Geometry check sheet. Reference: the model listing, model coordinates, mm. Face numbers are marked on the shaded views. A direction names the side the tool comes from. Coordinates: 2 decimals unless noted, no trailing zeros. Write each loop counter-clockwise with the first axis right and the second up, starting at its lowest first coordinate (ties: lowest second). Pieces come first, ordered by that corner, then holes. Notation, with made-up numbers: (-28, 45) - (-3, 45) arc R31 cw to (-3, 83) - close; hole circle Ø8 at (35.25, 49.25). An arc over 180 degrees is marked (long way). Answer as a JSON object with one key per item and string values. Group by question number.
from build123d import *

# Parameters (mm, degrees)
SKETCH1_R               = 5
BOSS_EXTRUDE1_DEPTH     = 22
FILLET1_R               = 1
FILLET2_R               = 10
SKETCH3_W               = 18
SKETCH3_H               = 10
CUT_EXTRUDE2_DEPTH      = 45
CUT_EXTRUDE2_DEPTH_BACK = 46


with BuildPart() as part:
    # Sketch1 → Boss-Extrude1 (new body)
    with BuildSketch(Plane(origin=(0, 0, 0), x_dir=(1, 0, 0), z_dir=(0, 1, 0))):
        with BuildLine():
            Line((44, 17), (35, 26))
            Line((35, 26), (25, 26))
            Line((25, 26), (5, 20.641016151))
            Line((5, 20.641016151), (-15, 26))
            Line((-15, 26), (-25, 26))
            Line((-25, 26), (-44.391127187, -9.608765584))
            ThreePointArc((-44.391127187, -9.608765584), (-38.766232585, -7.154608585), (-35, -12))
            ThreePointArc((-35, -12), (-36.464466094, -15.535533906), (-40, -17))
            Line((-40, -17), (-26.36195996, -17))
            Line((-26.36195996, -17), (-13.660254038, 5))
            ThreePointArc((-13.660254038, 5), (-10, 8.660254038), (-5, 10))
            Line((-5, 10), (5, 10))
            ThreePointArc((5, 10), (10, 8.660254038), (13.660254038, 5))
            Line((13.660254038, 5), (25.784609691, -16))
            Line((25.784609691, -16), (44, -16))
            Line((44, -16), (44, -4))
            Line((44, -4), (39.5, 0.5))
            Line((39.5, 0.5), (44, 5))
            Line((44, 5), (44, 17))
        make_face()
        with Locations((-40, -12)):
            Circle(SKETCH1_R)
    extrude(amount=BOSS_EXTRUDE1_DEPTH)

    # Fillet1
    fillet1_edges = [part.edges().sort_by_distance(p)[0] for p in [
        (-25, 11, -26),
        (-15, 11, -26),
        (25, 11, -26),
        (35, 11, -26),
        (44, 11, -17),
        (44, 11, -5),
        (39.5, 11, -0.5),
        (44, 11, 4),
        (44, 11, 16),
    ]]
    fillet(fillet1_edges, radius=FILLET1_R)

    # Fillet2
    fillet2_edges = [part.edges().sort_by_distance(p)[0] for p in [
        (-26.36195996, 11, 17),
        (5, 11, -20.641016151),
        (25.784609691, 11, 16),
    ]]
    fillet(fillet2_edges, radius=FILLET2_R)

    # Sketch3 → Cut-Extrude2 (cut, two sides)
    with BuildSketch(Plane(origin=(0, 0, 0), x_dir=(0, 0, -1), z_dir=(1, 0, 0))) as cut_extrude2_sk:
        Polygon((-9, 22), (-9, 31.2), (-17, 31.2), (-17, 4), (-13, 22), align=None)
        with Locations((0, 26.2)):
            Rectangle(SKETCH3_W, SKETCH3_H)
        Polygon((26, 31.2), (9, 31.2), (9, 22), (13, 22), (26, 4), align=None)
        with BuildLine():
            Line((11.743443525, 15.2), (-9.389141968, 15.2))
            Line((-9.389141968, 15.2), (-11.066743885, 7.650791373))
            ThreePointArc((-11.066743885, 7.650791373), (-10.478308141, 5.122817819), (-8.138182705, 4))
            Line((-8.138182705, 4), (13.965065195, 4))
            ThreePointArc((13.965065195, 4), (16.636152519, 5.634242881), (16.39710288, 8.756471662))
            Line((16.39710288, 8.756471662), (11.743443525, 15.2))
        make_face()
    extrude(amount=CUT_EXTRUDE2_DEPTH, mode=Mode.SUBTRACT)
    extrude(cut_extrude2_sk.sketch, amount=-CUT_EXTRUDE2_DEPTH_BACK, mode=Mode.SUBTRACT)


solid = part.part
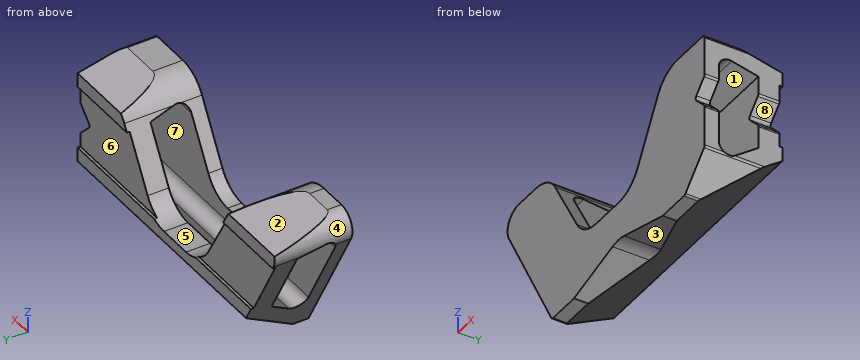
(1) Draft check along Z on the marked faces 1, 2 and 3. Enter one of: +Z half, -Z half, draft (parallel to the pull), parting line (faces both ways), or undercut.
(2) Section check D-D (z = 2). Record the cut outline in (x, y).
(3) Section check B-B (z = -7). Record the cut outline in (x, y), and give its area (3 significant figures).
(4) Material ranges on L1, parallel to Y at x = 32, z = -4; L2, parallel to X at y = 16.75, z = -9; L3, parallel to X at y = 16.25, z = 0, recorded low to high. Write a range as [from, to].
(5) Section check C-C (x = 17). Record the cut outline in (y, z).
(6) Set-up check for the marked faces 4, 5, 6, 7 and 8: record each of +Z, -Z, +X, -X, +Y, -Y from which the full face is reachable in a straight line by a thin tool's end or side.
(7) Gauge pin test, flat ends, axial feed: pin 1 (9.5 mm diameter, centred on x = 36.5, y = 3.5, fed in from +Z); pin 2 (0.9 mm diameter, centred on x = 28, y = 21.5, fed in from +Z); pin 3 (2 mm diameter, centred on y = 14.5, z = 2.5, fed in from +X). Record the tip position at first contact, or that the pin passes through.
Conclusion:
{
 "1": {"face 1": "undercut", "face 2": "+Z half", "face 3": "-Z half"},
 "2": {"outline": "(-40.25, 0) - (-17.7, 0) - (-17.7, 4) - (-40.25, 4) - close; (-40.25, 15.2) - (-17.7, 15.2) - (-17.7, 21.2) - (-40.25, 21.2) - close; (17.7, 0) - (42, 0) - (42, 4) - (17.7, 4) - close; (17.7, 15.2) - (42, 15.2) - (42, 21.2) - (17.7, 21.2) - close"},
 "3": {"outline": "(-35.35, 0) - (-12.14, 0) - (-12.14, 4) - (-35.35, 4) - close; (-35.35, 15.2) - (-12.14, 15.2) - (-12.14, 21.2) - (-35.35, 21.2) - close; (12.14, 0) - (44, 0) - (44, 4) - (12.14, 4) - close; (12.14, 15.2) - (44, 15.2) - (44, 21.2) - (12.14, 21.2) - close", "area": "551 mm^2"},
 "4": {"L1": "y = [0, 4], [15.2, 21.2]", "L2": "x = [-34.26, -9.36], [9.36, 44]", "L3": "x = [-39.16, -16.55], [16.55, 40.05]"},
 "5": {"outline": "(0, -23.86) - (6.97, -23.86) - (22, -13) - (22, -9) - (21.2, -9) - (21.2, 0.78) - (15.2, 0.78) - (15.2, -11.74) - (8.76, -16.4) arc R3 cw to (4, -13.97) - (4, 0.78) - (0, 0.78) - close"},
 "6": {"face 4": "-X, +Y, -Y", "face 5": "+Z, +Y, -Y", "face 6": "+X, -X, +Y", "face 7": "+X, -X", "face 8": "+X, +Y, -Y"},
 "7": {"pin 1": "stops at z = 16", "pin 2": "stops at z = 13.21", "pin 3": "stops at x = 43.21"}
}
